Input: dimensioned drawing with shaded views. Units: mm. Origin: part minimum x, y, z. Coordinates: 2 decimals unless noted, no trailing zeros. Order: outer loops, then holes, each group sorted by start corner. A loop starts at its lowest first (then second) coordinate and runs counter-clockwise, first axis right, second up.
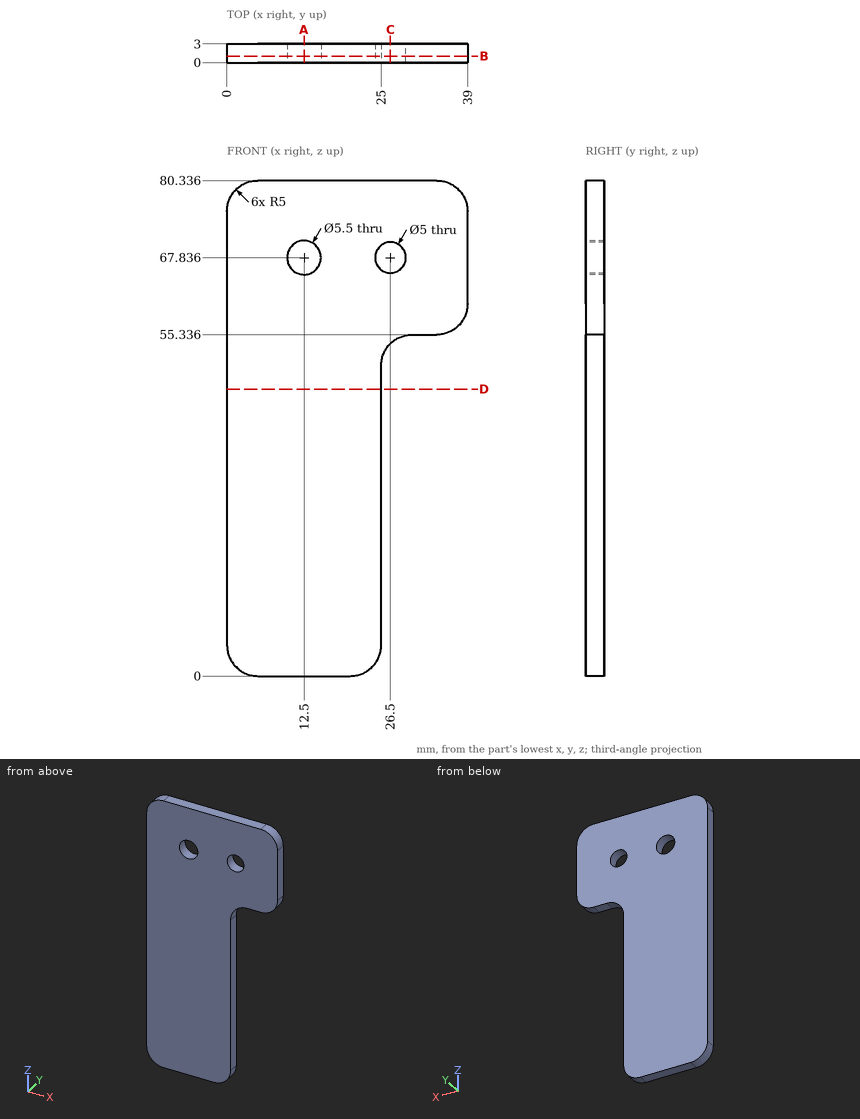
1. Section query D-D, the plane z = 46.5. Output: boundary loops of the cut face in (x, y), plus the area to 3 significant figures.
2. Section query B-B, the plane y = 1.05. Output: boundary loops of the cut face in (x, z), plus the area to 3 significant figures.
3. Section query A-A, the plane x = 12.5. Output: boundary loops of the cut face in (y, z).
4. Material intervals for line 1 along Z through (x, y) = (12.5, 1.15); line 2 along Z through (x, y) = (33.5, 1.9); line 3 along X through (y, z) = (0.7, 69), sorted ascending.
5. Section query C-C, the plane x = 26.5. Output: boundary loops of the cut face in (y, z), plus the area to 3 significant figures.
Answer key:
1. outline: (0, 0) - (25, 0) - (25, 3) - (0, 3) - close
1. area: 75.0 mm2
2. outline: (0, 5) arc R5 ccw to (5, 0) - (20, 0) arc R5 ccw to (25, 5) - (25, 50.34) arc R5 cw to (30, 55.34) - (34, 55.34) arc R5 ccw to (39, 60.34) - (39, 75.34) arc R5 ccw to (34, 80.34) - (5, 80.34) arc R5 ccw to (0, 75.34) - close; hole circle Ø5.5 at (12.5, 67.84); hole circle Ø5 at (26.5, 67.84)
2. area: 2,290 mm2
3. outline: (0, 0) - (3, 0) - (3, 65.09) - (0, 65.09) - close; (0, 70.59) - (3, 70.59) - (3, 80.34) - (0, 80.34) - close
4. line 1: z = 0 to 65.09, 70.59 to 80.34
4. line 2: z = 55.34 to 80.34
4. line 3: x = 0 to 10.01, 14.99 to 24.29, 28.71 to 39
5. outline: (0, 53.91) - (3, 53.91) - (3, 65.34) - (0, 65.34) - close; (0, 70.34) - (3, 70.34) - (3, 80.34) - (0, 80.34) - close
5. area: 64.3 mm2
